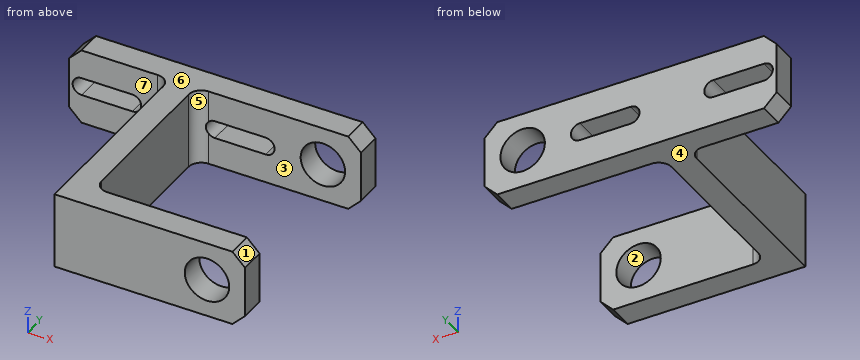
from build123d import *

# Parameters (mm, degrees)
BOSS_EXTRUDE1_DEPTH = 30
CHAMFER1_SIZE       = 10
CHAMFER2_SIZE       = 10
SKETCH2_R           = 17.5
CUT_EXTRUDE1_DEPTH  = 212
CUT_EXTRUDE2_DEPTH  = 111


with BuildPart() as part:
    # Sketch1 → Boss-Extrude1 (new, symmetric)
    with BuildSketch(Plane.XY):
        with BuildLine():
            Line((0, 150), (0, 0))
            Line((0, 0), (150, 0))
            Line((150, 0), (150, 20))
            Line((150, 20), (30, 20))
            ThreePointArc((30, 20), (22.928932188, 22.928932188), (20, 30))
            Line((20, 30), (20, 150))
            ThreePointArc((20, 150), (22.928932188, 157.071067812), (30, 160))
            Line((30, 160), (150, 160))
            Line((150, 160), (150, 180))
            Line((150, 180), (-80, 180))
            Line((-80, 180), (-80, 160))
            Line((-80, 160), (-10, 160))
            ThreePointArc((-10, 160), (-2.928932188, 157.071067812), (0, 150))
        make_face()
    extrude(amount=BOSS_EXTRUDE1_DEPTH, both=True)

    # Chamfer1
    chamfer1_edges = [part.edges().sort_by_distance(p)[0] for p in [
        (150, 170, 30),
    ]]
    chamfer(chamfer1_edges, length=CHAMFER1_SIZE)

    # Chamfer2
    chamfer2_edges = [part.edges().sort_by_distance(p)[0] for p in [
        (-80, 170, 30),
        (150, 10, -30),
        (150, 170, -30),
        (-80, 170, -30),
        (150, 10, 30),
    ]]
    chamfer(chamfer2_edges, length=CHAMFER2_SIZE)

    # Sketch2 → Cut-Extrude1 (cut)
    with BuildSketch(Plane(origin=(0, 180, 0), x_dir=(1, 0, 0), z_dir=(0, 1, 0))):
        with BuildLine():
            ThreePointArc((-30, 7), (-23, 0), (-30, -7))
            Line((-30, -7), (-70, -7))
            ThreePointArc((-70, -7), (-77, 0), (-70, 7))
            Line((-70, 7), (-30, 7))
        make_face()
        with Locations(Location((120, 0, 0), (0, 0, 180))):
            Circle(SKETCH2_R)
    extrude(amount=-CUT_EXTRUDE1_DEPTH, mode=Mode.SUBTRACT)

    # Sketch4 → Cut-Extrude2 (cut)
    with BuildSketch(Plane(origin=(0, 180, 0), x_dir=(1, 0, 0), z_dir=(0, 1, 0))):
        with BuildLine():
            Line((75, 7), (35, 7))
            ThreePointArc((35, 7), (28, 0), (35, -7))
            Line((35, -7), (75, -7))
            ThreePointArc((75, -7), (82, 0), (75, 7))
        make_face()
    extrude(amount=-CUT_EXTRUDE2_DEPTH, mode=Mode.SUBTRACT)


solid = part.part
Check sheet for the modelled part. Datum: model origin and axes. Units: mm. Face numbers are marked on the shaded views. A direction names the side the tool comes from. Round coordinates to 2 decimals unless told otherwise and drop trailing zeros. Loops run counter-clockwise (first coordinate to the right, second up) from the corner with the lowest first, then second, coordinate; pieces in that order, holes last. Notation, with made-up numbers: (-6, -10.5) - (26, -10.5) arc R26 ccw to (26, 6.5) - close; hole circle Ø9 at (25, -23.5). An arc over 180 degrees is marked (long way). Answer as CSV lines item,"result". Start each with the question number.
Item 1: Section check C-C (x = -32.5). Record the boundary of the cut face in (y, z).
Item 2: Section check A-A (x = 120). Record the boundary of the cut face in (y, z).
Item 3: Set-up check for the marked faces 5, 6 and 7: record each of +Z, -Z, +X, -X, +Y, -Y from which the full face is reachable in a straight line by a thin tool's end or side.
Item 4: Release check for a two-part mould opening along Z. For the marked faces 1, 2, 3 and 4 record: +Z half, -Z half, draft (parallel to the pull), parting line (faces both ways), or undercut.
Item 5: Section check B-B (z = 0). Record the boundary of the cut face in (x, y).
Item 6: Section check D-D (z = -25.5). Record the boundary of the cut face in (x, y), and give its area (3 significant figures).
Item 7: Scan lines: line 1 (Y direction, x = 99.5, z = 6.5); line 2 (Z direction, x = 120, y = 10.25); line 3 (X direction, y = 143, z = -11). Record each from-to range of solid material in increasing order. Write a range as [from, to].
Item 8: Depth check by flat-ended pin: P1, Ø21, axis at x = 120, z = 0, coming from the -Y side; P2, Ø6, axis at y = 152, z = 15, coming from the +X side; P3, Ø10, axis at y = 97.5, z = 20, coming from the +X side; P4, Ø3, axis at y = 37, z = -15, coming from the -X side. Enter the tip coordinate at first touch or a pass-through.
Report:
1,outline,"(160, -30) - (180, -30) - (180, -7) - (160, -7) - close; (160, 7) - (180, 7) - (180, 30) - (160, 30) - close"
2,outline,"(0, -30) - (20, -30) - (20, -17.5) - (0, -17.5) - close; (0, 17.5) - (20, 17.5) - (20, 30) - (0, 30) - close; (160, -30) - (180, -30) - (180, -17.5) - (160, -17.5) - close; (160, 17.5) - (180, 17.5) - (180, 30) - (160, 30) - close"
3,face 5,"+Z, -Z, +X"
3,face 6,"+Z, +X, -X, +Y, -Y"
3,face 7,"+Z, -Z, -X, -Y"
4,face 1,"+Z half"
4,face 2,"undercut"
4,face 3,"draft"
4,face 4,"-Z half"
5,outline,"(-80, 160) - (-77, 160) - (-77, 180) - (-80, 180) - close; (-23, 160) - (-10, 160) arc R10 cw to (0, 150) - (0, 0) - (102.5, 0) - (102.5, 20) - (30, 20) arc R10 cw to (20, 30) - (20, 150) arc R10 cw to (28, 159.8) - (28, 180) - (-23, 180) - close; (82, 160) - (102.5, 160) - (102.5, 180) - (82, 180) - close; (137.5, 0) - (150, 0) - (150, 20) - (137.5, 20) - close; (137.5, 160) - (150, 160) - (150, 180) - (137.5, 180) - close"
6,outline,"(-74.5, 160) - (-10, 160) arc R10 cw to (0, 150) - (0, 0) - (144.5, 0) - (144.5, 20) - (30, 20) arc R10 cw to (20, 30) - (20, 150) arc R10 cw to (30, 160) - (144.5, 160) - (144.5, 180) - (-74.5, 180) - close"
6,area,"10,100 mm2"
7,line 1,"y = [0, 20], [160, 180]"
7,line 2,"z = [-30, -17.5], [17.5, 30]"
7,line 3,"x = [0, 20]"
8,P1,"passes through"
8,P2,"stops at x = 21.34"
8,P3,"stops at x = 20"
8,P4,"stops at x = 0"
